Here's how the part is built. I have some questions about the finished solid (model axes, mm). A direction names the side the tool comes from. Round coordinates to 2 decimals unless told otherwise and drop trailing zeros. Order: outer loops, then holes, each group sorted by start corner. A loop starts at its lowest first (then second) coordinate and runs counter-clockwise, first axis right, second up. Notation, with made-up numbers: (25, 34) -> (34, 34) arc R13 cw to (34, 58) -> close; hole circle Ø2 at (10.5, 65). An arc over 180 degrees is marked (long way). Answer in a Markdown table with one row per item.
```python
from build123d import *

# Parameters (mm, degrees)
F0_R       = 10.16
F1_DEPTH   = 40.2336
F2_R       = 10.16
F3_DEPTH   = 24.4602
F4_C1_SIZE = 3.302
F4_C2_SIZE = 3.302
F4_C3_SIZE = 3.302
F4_C4_SIZE = 3.302


with BuildPart() as f1:
    # F0 (on Top) → F1 (new body)
    with BuildSketch(Plane.XY):
        with BuildLine():
            Line((57.1919272622, 18.7764181619), (9.5121844836, 26.9452959039))
            ThreePointArc((9.5121844836, 26.9452959039), (23.3274655355, 16.5033322905), (28.575, 0))
            ThreePointArc((28.575, 0), (23.3274655355, -16.5033322905), (9.5121844836, -26.9452959039))
            Line((9.5121844836, -26.9452959039), (57.1919272622, -18.7764181619))
            ThreePointArc((57.1919272622, -18.7764181619), (73.025, 0), (57.1919272622, 18.7764181619))
        make_face()
        with Locations((53.975, 0)):
            Circle(F0_R, mode=Mode.SUBTRACT)
        with BuildLine():
            Line((9.5121844836, 26.9452959039), (0, 28.575))
            ThreePointArc((0, 28.575), (-28.575, 0), (0, -28.575))
            Line((0, -28.575), (9.5121844836, -26.9452959039))
            ThreePointArc((9.5121844836, -26.9452959039), (23.3274655355, -16.5033322905), (28.575, 0))
            ThreePointArc((28.575, 0), (23.3274655355, 16.5033322905), (9.5121844836, 26.9452959039))
        make_face()
        with BuildLine():
            ThreePointArc((13.7595011415, -3.8482183654), (-14.2865339733, 0.1661423458), (13.845272005, 3.5271942616))
            Line((13.845272005, 3.5271942616), (19.0572988585, 3.5271942616))
            Line((19.0572988585, 3.5271942616), (19.0572988585, -3.8482183654))
            Line((19.0572988585, -3.8482183654), (13.7595011415, -3.8482183654))
        make_face(mode=Mode.SUBTRACT)
    extrude(amount=F1_DEPTH)

    # F2 (on face) → F3 (cut)
    with BuildSketch(Plane.XY.offset(40.2336)):
        with BuildLine():
            Line((57.1919272622, 18.7764181619), (9.5121844836, 26.9452959039))
            ThreePointArc((9.5121844836, 26.9452959039), (23.3274655355, 16.5033322905), (28.575, 0))
            ThreePointArc((28.575, 0), (23.3274655355, -16.5033322905), (9.5121844836, -26.9452959039))
            Line((9.5121844836, -26.9452959039), (57.1919272622, -18.7764181619))
            ThreePointArc((57.1919272622, -18.7764181619), (73.025, 0), (57.1919272622, 18.7764181619))
        make_face()
        with Locations((53.975, 0)):
            Circle(F2_R, mode=Mode.SUBTRACT)
    extrude(amount=-F3_DEPTH, mode=Mode.SUBTRACT)

    # F4: chamfer of 3.302 on 4 edges, made by hand

    # F4_c1
    f4_c1_edges = [f1.edges().sort_by_distance(p)[0] for p in [
        (4.7560922418, 27.760147952, 40.2336),
    ]]
    chamfer(f4_c1_edges, length=F4_C1_SIZE)

    # F4_c2
    f4_c2_edges = [f1.edges().sort_by_distance(p)[0] for p in [
        (4.7560922418, -27.760147952, 40.2336),
    ]]
    chamfer(f4_c2_edges, length=F4_C2_SIZE)

    # F4_c3
    f4_c3_edges = [f1.edges().sort_by_distance(p)[0] for p in [
        (-28.575, 0, 40.2336),
    ]]
    chamfer(f4_c3_edges, length=F4_C3_SIZE)

    # F4_c4
    f4_c4_edges = [f1.edges().sort_by_distance(p)[0] for p in [
        (28.575, 0, 40.2336),
    ]]
    chamfer(f4_c4_edges, length=F4_C4_SIZE)


solid = f1.part
```
1. Suppose I cut it at B-B on x = 49.5. Write out the boundary of the cut face in (y, z), then the cut area to 3 significant figures.
Numbers:
| item | result |
|---|---|
| outline | (-20.09, 0) -> (-9.12, 0) -> (-9.12, 15.77) -> (-20.09, 15.77) -> close; (9.12, 0) -> (20.09, 0) -> (20.09, 15.77) -> (9.12, 15.77) -> close |
| area | 346 mm2 |
2. For pin 1 Ø4 at (x, z) = (28, 13) entering from +Y; pin 2 Ø1.5 at (y, z) = (-10.5, 9) entering from +X; pin 3 Ø2.5 at (x, z) = (16.5, 20) entering from -Y; pin 4 Ø16.5 at (x, y) = (53.975, 0) entering from -Z, each with a flat end and sliding along its axis, tell me the tip position at first contact or that it passes through.
Numbers:
| item | result |
|---|---|
| pin 1 | stops at y = 24.12 |
| pin 2 | stops at x = 70.34 |
| pin 3 | stops at y = -24.17 |
| pin 4 | passes through |
3. For faces 1 (the face through (16, -3.848, 20)), 2 (the face through (22, 0, 0)), which set-ups out of +Z, -Z, +X, -X, +Y, -Y let a thin tool reach every point of the face, with its end or its side?
Numbers:
| item | result |
|---|---|
| face 1 | +Z, -Z |
| face 2 | -Z, +X, -X, +Y, -Y |
4. Please list where these lines run through material, in increasing order: line 1 along Y through (x, z) = (0, 22.5) (1 decimal); line 2 along X through (y, z) = (8, 7.5); line 3 along Z through (x, y) = (45.5, 15.5).
Numbers:
| item | result |
|---|---|
| line 1 | y = -28.6 to -14.3, 14.3 to 28.6 |
| line 2 | x = -27.43 to -11.84, 11.84 to 47.71, 60.24 to 71.26 |
| line 3 | z = 0 to 15.77 |
5. We'd pull the mould along Y, two halves only. Please class faces 3 (the face through (43.825, 0.447, 7.776)), 4 (the face through (-28.57, 0.63, 18.21)), 5 (the face through (4.54, 26.099, 38.606)): released by +Y, released by -Y, zero draft, split by the parting line, or undercut.
Numbers:
| item | result |
|---|---|
| face 3 | undercut |
| face 4 | split by the parting line |
| face 5 | released by +Y |
6. Suppose I cut it at C-C on z = 5. State how many separate pieces and enclosed holes the cut face has, then the cut area to 3 significant figures.
Numbers:
| item | result |
|---|---|
| separate pieces | 1 |
| enclosed holes | 2 |
| area | 3,440 mm2 |
